Model file for the job. Use its own axes, mm. A direction names the side the tool comes from. Give positions to 0.01 mm unless a question says otherwise; leave off trailing zeros. Loops run counter-clockwise (first coordinate to the right, second up) from the corner with the lowest first, then second, coordinate; pieces in that order, holes last. Notation, with made-up numbers: (88.25, 79.5) - (127.25, 79.5) arc R26 ccw to (127.25, 114.5) - close; hole circle Ø8 at (21, 78). An arc over 180 degrees is marked (long way). Use a Markdown table: item, result.
from build123d import *

# Parameters (mm, degrees)
SKETCH1_R           = 1.5
BOSS_EXTRUDE1_DEPTH = 3.175
SKETCH2_R           = 2.2479
CUT_EXTRUDE1_DEPTH  = 4.175
FILLET1_R           = 2.54


with BuildPart() as part:
    # Sketch1 → Boss-Extrude1 (new body)
    with BuildSketch(Plane(origin=(0, 0, 0), x_dir=(1, 0, 0), z_dir=(0, 1, 0))):
        Polygon((14.664696837, 25.4), (-14.664696837, -25.4), (10.500295474, -25.4), (1.583973528, -9.956477372), (21.997045256, 25.4), align=None)
        with Locations((-8.432200682, -22.225)):
            Circle(SKETCH1_R, mode=Mode.SUBTRACT)
        with Locations((4.267799318, -22.225)):
            Circle(SKETCH1_R, mode=Mode.SUBTRACT)
    extrude(amount=BOSS_EXTRUDE1_DEPTH)

    # Sketch2 → Cut-Extrude1 (cut, through all)
    with BuildSketch(Plane(origin=(0, 3.175, 0), x_dir=(1, 0, 0), z_dir=(0, 1, 0))):
        with Locations((15.826827494, 21.062869343)):
            Circle(SKETCH2_R)
    extrude(amount=-CUT_EXTRUDE1_DEPTH, mode=Mode.SUBTRACT)

    # Fillet1
    fillet1_edges = [part.edges().sort_by_distance(p)[0] for p in [
        (-14.664696837, 1.5875, 25.4),
        (14.664696837, 1.5875, -25.4),
        (21.997045256, 1.5875, -25.4),
        (1.583973528, 1.5875, 9.956477372),
        (10.500295474, 1.5875, 25.4),
    ]]
    fillet(fillet1_edges, radius=FILLET1_R)


solid = part.part
(1) Slice it at C-C, the plane x = 0. Write the cut outline in (y, z) (3 decimals), plus the area to 3 significant figures.
Computed:
| item | result |
|---|---|
| outline | (0, 0) - (3.175, 0) - (3.175, 25.4) - (0, 25.4) - close |
| area | 80.6 mm² |
(2) Drill centre lines: probe 1 along X at (y, z) = (0.7, 21); probe 2 along Z at (x, y) = (5.5, 2); probe 3 along Z at (x, y) = (-8, 1.3). Where is each one in solid material? Low to high. Write a range as [from, to].
Computed:
| item | result |
|---|---|
| probe 1 | [-12.12, -9.3], [-7.57, 3.4], [5.13, 7.96] |
| probe 2 | [-9.53, 3.17], [16.74, 21.37], [23.08, 25.4] |
| probe 3 | [13.86, 20.79], [23.66, 25.4] |
(3) Slice it at A-A, the plane x = 17. Write the cut outline in (y, z) (3 decimals).
Computed:
| item | result |
|---|---|
| outline | (0, -25.4) - (3.175, -25.4) - (3.175, -22.98) - (0, -22.98) - close; (0, -19.145) - (3.175, -19.145) - (3.175, -16.745) - (0, -16.745) - close |
(4) Mould opens along Z. For faces 3 (the cylindrical face through (15.34, 1.61, -18.87)), 4 (the flat face through (0.92, 1.57, -1.59)), 5 (the flat face through (-2, 2, 25.4)), 6 (the cylindrical face through (-12.48, 1.61, 24.1)) say: pulls with the +Z half, pulls with the -Z half, needs draft (parallel to the pull), parting line crosses it, or undercut.
Computed:
| item | result |
|---|---|
| face 3 | undercut |
| face 4 | pulls with the -Z half |
| face 5 | pulls with the +Z half |
| face 6 | parting line crosses it |
(5) Slice it at D-D, the plane z = 0.5. Write the cut outline in (x, y) (3 decimals), plus the area to 3 significant figures.
Computed:
| item | result |
|---|---|
| outline | (-0.289, 0) - (7.044, 0) - (7.044, 3.175) - (-0.289, 3.175) - close |
| area | 23.3 mm² |
(6) Pin check, flat tips, straight feed: P1, Ø4, axis at x = 10.5, z = -6.5, coming from the -Y side; P2, Ø1, axis at x = 6, y = 0.5, coming from the -Z side. Stop position of each tip, or through.
Computed:
| item | result |
|---|---|
| P1 | y = 0 |
| P2 | z = -11.26 |
(7) Slice it at B-B, the plane y = 1.2. Write the cut outline in (x, z) (3 decimals), plus the area to 3 significant figures.
Computed:
| item | result |
|---|---|
| outline | (-12.465, 21.59) - (13.931, -24.13) arc R2.54 ccw to (16.131, -25.4) - (17.598, -25.4) arc R2.54 ccw to (19.797, -21.59) - (2.317, 8.686) arc R2.54 cw to (2.317, 11.226) - (8.301, 21.59) arc R2.54 ccw to (6.101, 25.4) - (-10.265, 25.4) arc R2.54 ccw to start; hole circle Ø3 at (-8.432, 22.225); hole circle Ø3 at (4.268, 22.225); hole circle Ø4.496 at (15.827, -21.063) |
| area | 467 mm² |
(8) 3-axis set-ups, long thin cutter, end or side, ignore diameter. For faces 1 (the flat face through (10.935, 1.565, -6.24)), 2 (the flat face through (2, 3.175, 7)): which of +Z, -Z, +X, -X, +Y, -Y reach the whole face in a straight line?
Computed:
| item | result |
|---|---|
| face 1 | +X, +Y, -Y |
| face 2 | +Z, -Z, +X, -X, +Y |
